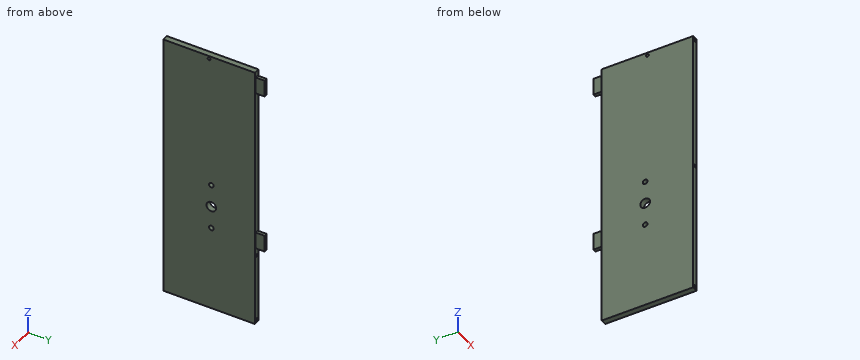
Autodesk Inventor part; units mm, degrees
ref_plane "YZ Plane" through (0, 0, 0) normal (1, 0, 0) x (0, 1, 0)
ref_plane "XZ Plane" through (0, 0, 0) normal (0, 1, 0) x (-1, 0, 0)
ref_plane "XY Plane" through (0, 0, 0) normal (0, 0, 1) x (1, 0, 0)
sketch "Esquisse1" plane through (0, 0, 0) normal (1, 0, 0) x (0, 1, 0)
  line L0 (0, 0) -> (80, 0)
  line L1 (80, 0) -> (80, -200)
  line L2 (80, -200) -> (0, -200)
  line L3 (0, -200) -> (0, 0)
  dimension "d0" = 80
  dimension "d1" = 200
extrude "Extrusion1" add sketch "Esquisse1" along normal blind 5
sketch "Esquisse7" plane through (5, 0, 0) normal (1, 0, 0) x (0, 0, -1)
  line L0 (0, 0) -> (100, 0)
  line L1 (0, 0) -> (200, 0)
  line L2 (100, 0) -> (180, 0) construction
  line L3 (100, 80) -> (100, 10)
  line L4 (100, 80) -> (170, 80) construction
  line L5 (120, 42) -> (80, 42)
  dimension "d50" = 100
  dimension "d54" = 90
  dimension "d80" = 40
hole "Perçage6" at (5, 42, -120) at (5, 42, -80) direction (-1, 0, 0) diameter 4.134 end through all
sketch "Esquisse8" plane through (5, 0, 0) normal (1, 0, 0) x (0, 0, -1)
  circle A0 centre (80, 42) radius 2.067
  line L0 (80, 42) -> (100, 42)
  point P0 (0, 0)
hole "Perçage7" at (5, 42, -100) direction (-1, 0, 0) diameter 8.5 end through all
sketch "Esquisse9" plane through (0, 0, 0) normal (0, 0, 1) x (1, 0, 0)
  line L0 (0, 80) -> (0, 0)
  line L1 (0, 0) -> (5, 0)
  line L2 (5, 80) -> (5, 0)
  line L3 (0, 80) -> (5, 80)
extrude "Extrusion2" add sketch "Esquisse9" along normal blind 40
sketch "Esquisse5" plane through (0, 80, 0) normal (0, 1, 0) x (1, 0, 0)
  line L0 (0, 0) -> (5, 0)
  line L1 (2.5, 0) -> (5, 0) construction
  line L2 (0, 200) -> (0, 0)
  line L3 (0, 200) -> (5, 200)
  line L4 (0, 200) -> (0, 132.45)
  line L5 (0, 132.45) -> (2.5, 132.45)
  point P0 (2.5, 197.5)
  point P1 (0, -40)
  point P2 (2.5, 200)
  dimension "d84" = 2.5
  dimension "d85" = 2.5
  dimension "d86" = 67.55
hole "Perçage4" at (2.5, 80, -197.5) at (2.5, 80, -132.45) direction (0, -1, 0) diameter 2.459 depth 15
sketch "Esquisse4" plane through (0, 0, -200) normal (0, -1, 0) x (1, 0, 0)
  line L0 (0, 0) -> (0, 200)
  line L1 (5, 200) -> (5, 0)
  line L2 (5, 240) -> (0, 240)
  line L3 (0, 240) -> (2.5, 240)
  line L4 (2.5, 237.5) -> (2.5, 240)
  line L5 (0, 240) -> (0, 120)
  line L6 (0, 0) -> (5, 0)
  line L7 (0, 120) -> (2.5, 120)
  point P0 (2.5, 2.5)
  point P1 (2.5, 0)
  dimension "d87" = 120
  dimension "d88" = 2.5
  dimension "d89" = 2.5
hole "Perçage3" at (2.5, 0, -197.5) at (2.5, 0, 37.5) at (2.5, 0, -80) direction (0, 1, 0) diameter 2.459 depth 15
sketch "Esquisse3" plane through (5, 0, 0) normal (1, 0, 0) x (0, 0, -1)
  line L0 (0, 0) -> (200, 0)
  line L1 (-39.8826, 0) -> (-37.3826, 0)
  line L2 (-37.3826, 0) -> (-37.3826, 40)
  point P0 (197.5, 40)
  dimension "d90" = 2.5
  dimension "d91" = 40
hole "Perçage2" at (5, 40, -197.5) at (5, 40, 37.3826) direction (-1, 0, 0) diameter 2.459 end through all
sketch "Esquisse10" plane through (0, 80, -200) normal (0, 1, 0) x (1, 0, 0)
  line L0 (5, -240) -> (0, -240)
  line L1 (2.5, -240) -> (2.5, -234.9)
  line L2 (2.5, -234.9) -> (3.9, -234.9)
  line L3 (2.5, -234.9) -> (1.1, -234.9)
  line L4 (1.1, -234.9) -> (1.1, -220.1)
  line L5 (1.1, -220.1) -> (3.9, -220.1)
  line L6 (3.9, -220.1) -> (3.9, -234.9)
  line L7 (0, -240) -> (0, -89.9)
  line L8 (0, 0) -> (0, -240)
  line L9 (0, -89.9) -> (1.1, -89.9)
  line L10 (1.1, -89.9) -> (3.9, -89.9)
  line L11 (3.9, -89.9) -> (3.9, -75.1)
  line L12 (3.9, -75.1) -> (1.1, -75.1)
  line L13 (1.1, -75.1) -> (1.1, -89.9)
  point P0 (0, -200)
  dimension "d92" = 5.1
  dimension "d93" = 1.4
  dimension "d94" = 1.4
  dimension "d95" = 14.8
  dimension "d96" = 150.1
  dimension "d97" = 1.1
  dimension "d98" = 14.8
  dimension "d99" = 2.8
extrude "Extrusion3" add sketch "Esquisse10" along normal blind 8
sketch "Esquisse11" plane through (5, 0, 0) normal (1, 0, 0) x (0, 0, -1)
  line L0 (200, 80) -> (-40, 80)
  line L1 (200, 0) -> (-40, 0)
  line L2 (200, 80) -> (195, 80)
  line L3 (195, 80) -> (195, 0)
  line L4 (195, 0) -> (200, 0)
  line L5 (200, 0) -> (200, 80)
  point P0 (0, 0)
  dimension "d102" = 5
extrude "Extrusion4" cut sketch "Esquisse11" against normal blind 8
sketch "Esquisse12" plane through (0, 80, 40) normal (0, 1, 0) x (1, 0, 0)
  line L0 (0, 235) -> (0, 0)
  line L1 (0, 235) -> (2.5, 235)
  line L2 (0, 235) -> (5, 235)
  line L3 (2.5, 235) -> (2.5, 232.5)
  point P0 (0, 40)
  dimension "d105" = 2.5
  dimension "d106" = 2.5
hole "Perçage8" at (2.5, 80, -192.5) direction (0, -1, 0) diameter 2.459 depth 15
sketch "Esquisse13" plane through (0, 0, 40) normal (0, -1, 0) x (1, 0, 0)
  line L0 (0, -235) -> (0, 0)
  line L1 (0, -235) -> (2.5, -235)
  line L2 (5, -235) -> (0, -235)
  circle A0 centre (2.5, -232.5) radius 1.2295
  point P0 (0, -40)
hole "Perçage9" at (2.5, 0, -192.5) direction (0, 1, 0) diameter 2.459 depth 15
properties part number "chassis_côté"
Geometry: final body of the model. Coordinates: model frame, mm. Round coordinates to 2 decimals unless told otherwise and drop trailing zeros. Order: outer loops, then holes, each group sorted by start corner. A loop starts at its lowest first (then second) coordinate and runs counter-clockwise, first axis right, second up. Notation, with made-up numbers: M 36.5,-2.5 L 84.5,-2.5 A15 ccw 84.5,4.5 Z; hole C 10,17.5 d8. An arc over 180 degrees is marked long. Use one line per item in the form item = value. Start each with the question number.
Q1. Cut plane A-A (z = -100). Return loops of the section in (x, y), and give its area (4 significant figures).
Q2. Material intervals for line 1 (Z direction, x = 3.75, y = 42); line 2 (Z direction, x = 2.25, y = 78.5); line 3 (X direction, y = 10.75, z = 37.5), sorted ascending. Write a range as [from, to].
Q3. Pin query (flat end, axial travel): pin 1 Ø2.5 at (y, z) = (85.5, 28.5) entering from -X; pin 2 Ø0.7 at (x, z) = (2.5, -79.5) entering from -Y; pin 3 Ø2 at (x, y) = (3, 86) entering from +Z. Return the tip coordinate at first contact, or that it passes through.
Q4. Cut plane B-B (z = -137). Return loops of the section in (x, y), and give its area (3 significant figures).
Geometry results:
q1.outline = M 0,0 L 5,0 L 5,37.75 L 0,37.75 Z; M 0,46.25 L 5,46.25 L 5,80 L 0,80 Z
q1.area = 357.5 mm^2
q2.line_1 = [-195, -122.07], [-117.93, -104.25], [-95.75, -82.07], [-77.93, 40]
q2.line_2 = [-195, -193.7], [-191.3, -133.65], [-131.25, 40]
q2.line_3 = [0, 1.27], [3.73, 5]
q3.pin_1 = 1.1
q3.pin_2 = 15
q3.pin_3 = 34.9
q4.outline = M 0,0 L 5,0 L 5,80 L 0,80 Z
q4.area = 400 mm^2
